Could you check a few things on this model? Use its own coordinates, in mm. Face numbers are marked on the shaded views. Give positions to 0.01 mm unless a question says otherwise; leave off trailing zeros. Loops run counter-clockwise (first coordinate to the right, second up) from the corner with the lowest first, then second, coordinate; pieces in that order, holes last. Notation, with made-up numbers: M 57.5,-8 L 106.5,-8 A13 cw 106.5,13 Z; hole C 70,49.25 d8. An arc over 180 degrees is marked long. Write each question's results on one line, items separated by ' | '. Start each with the question number.
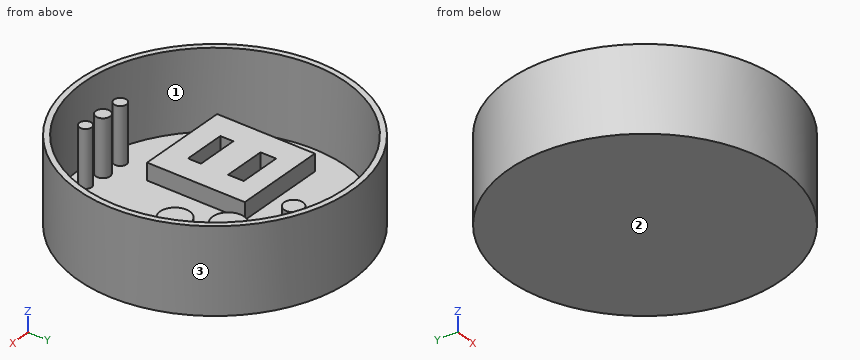
from build123d import *

# Parameters (mm, degrees)
F0_R     = 121.822916
F1_DEPTH = 75
F2_T     = -5
F3_R     = 8.352587
F3_R_2   = 13.960052
F3_R_3   = 13.177503
F3_R_4   = 5.384974
F3_R_5   = 6.304301
F3_R_6   = 5.548783
F4_DEPTH = 50
F5_W     = 81.67348
F5_H     = 87.06702
F5_W_2   = 37.754722
F5_H_2   = 11.557571
F5_H_3   = 13.869084
F6_DEPTH = 15


with BuildPart() as f1:
    # F0 (on Top) → F1 (new body)
    with BuildSketch(Plane.XY):
        Circle(F0_R)
    extrude(amount=F1_DEPTH)

    # F2
    f2_openings = [f1.faces().sort_by_distance(p)[0] for p in [
        (0, 0, 75),
    ]]
    offset(amount=F2_T, openings=f2_openings)

    # F3 (on face) → F4 (join)
    with BuildSketch(Plane.XY.offset(5)):
        with Locations((16.062267, 82.355626)):
            Circle(F3_R)
        with Locations((61.912745, 59.28437)):
            Circle(F3_R_2)
        with Locations((79.143174, 24.823505)):
            Circle(F3_R_3)
        with Locations((19.566761, -100.462183)):
            Circle(F3_R_4)
        with Locations((0, -99.878103)):
            Circle(F3_R_5)
        with Locations((-19.858804, -99.586062)):
            Circle(F3_R_6)
    extrude(amount=F4_DEPTH)

    # F5 (on face) → F6 (join)
    with BuildSketch(Plane.XY.offset(5)):
        with Locations((-52.394312, -25.811905)):
            Rectangle(F5_W, F5_H)
        with Locations((-52.394312, -43.918762)):
            Rectangle(F5_W_2, F5_H_2, mode=Mode.SUBTRACT)
        with Locations((-52.394312, -6.934542)):
            Rectangle(F5_W_2, F5_H_3, mode=Mode.SUBTRACT)
    extrude(amount=F6_DEPTH)


solid = f1.part
1) If we section it at D-D on x = -106: Write out the boundary of the cut face in (y, z).
2) Thinking about a two-plate mould opening in X: for the marked faces 1, 2 and 3, which applies, pulls with the +X half, pulls with the -X half, needs draft (parallel to the pull), parting line crosses it, or undercut?
3) If we section it at A-A on z = 42: Write out the boundary of the cut face in (x, y) (1 decimal).
4) If we section it at C-C on y = -86.5: Write out the boundary of the cut face in (x, z).
5) Please list where these lines run through material, in increasing order: line 1 (Y direction, x = 0, z = 24); line 2 (X direction, y = 25.5, z = 6.5); line 3 (Y direction, x = 15, z = 48). Write a range as from..to.
6) If we section it at B-B on x = 0: Write out the boundary of the cut face in (y, z), plus the area to 3 significant figures.
7) I'm going to push flat-ended pins straight in: P1, Ø5, axis at x = 44.5, y = -8, coming from the +Z side; P2, Ø13.5, axis at x = 18, y = 79, coming from the +Z side; P3, Ø16.5, axis at x = -59.5, z = 14, coming from the +Y side. Where does each tip first touch, or does it pass through?
Calculated:
1) outline: M -60.04,0 L 60.04,0 L 60.04,75 L 49.11,75 L 49.11,5 L -49.11,5 L -49.11,75 L -60.04,75 Z
2) face 1: undercut | face 2: needs draft | face 3: parting line crosses it
3) outline: C 0,0 d243.6; C -19.9,-99.6 d11.1; C 0,-99.9 d12.6; C 16.1,82.4 d16.7; C 19.6,-100.5 d10.8; C 61.9,59.3 d27.9; C 79.1,24.8 d26.4; hole C 0,0 d233.6
4) outline: M -85.78,0 L 85.78,0 L 85.78,75 L 78.52,75 L 78.52,5 L -78.52,5 L -78.52,75 L -85.78,75 Z
5) line 1: y = -121.82..-116.82, -106.18..-93.57, 116.82..121.82 | line 2: x = -119.12..-114.01, 65.98..92.3, 114.01..119.12 | line 3: y = -120.9..-115.86, -103.32..-97.61, 74.07..90.64, 115.86..120.9
6) outline: M -121.82,0 L 121.82,0 L 121.82,75 L 116.82,75 L 116.82,5 L -93.57,5 L -93.57,55 L -106.18,55 L -106.18,5 L -116.82,5 L -116.82,75 L -121.82,75 Z | area: 2,550 mm2
7) P1: stops at z = 5 | P2: stops at z = 55 | P3: stops at y = 110.52
